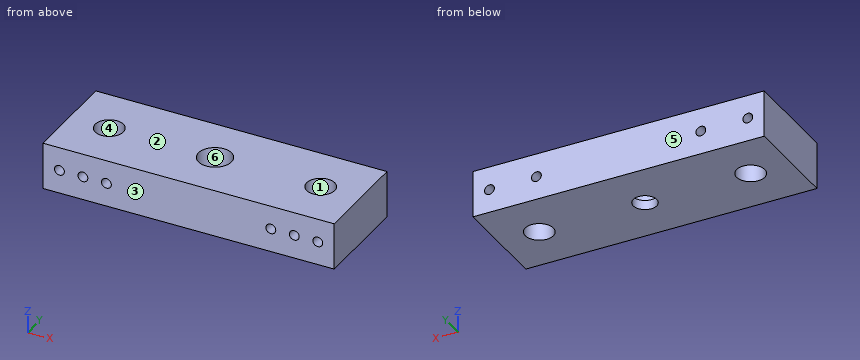
```python
from build123d import *

# Parameters (mm, degrees)
SKETCH1_W           = 124
SKETCH1_H           = 42.5
SKETCH1_R           = 6
SKETCH1_R_2         = 5
BOSS_EXTRUDE1_DEPTH = 20
CUT_EXTRUDE1_REACH  = 44.5
SKETCH2_R           = 2.1
SKETCH3_R           = 7.05
CUT_EXTRUDE2_DEPTH  = 16


with BuildPart() as part:
    # Sketch1 → Boss-Extrude1 (new body)
    with BuildSketch(Plane.XY):
        with Locations((62, 21.25)):
            Rectangle(SKETCH1_W, SKETCH1_H)
        with Locations((17, 21.25)):
            Circle(SKETCH1_R, mode=Mode.SUBTRACT)
        with Locations((107, 21.25)):
            Circle(SKETCH1_R, mode=Mode.SUBTRACT)
        with Locations((62, 21.25)):
            Circle(SKETCH1_R_2, mode=Mode.SUBTRACT)
    extrude(amount=BOSS_EXTRUDE1_DEPTH)

    # Sketch2 → Cut-Extrude1 (cut, up to next)
    with BuildSketch(Plane.XZ, mode=Mode.PRIVATE) as cut_extrude1_sk1:
        with Locations((7, 10)):
            Circle(SKETCH2_R)
    cut_extrude1_tool1 = extrude(cut_extrude1_sk1.sketch, amount=-CUT_EXTRUDE1_REACH, mode=Mode.PRIVATE) & part.part
    add(cut_extrude1_tool1.solids().sort_by_distance((7, 0, 10))[0], mode=Mode.SUBTRACT)
    # Sketch2 → Cut-Extrude1 (cut, up to next)
    with BuildSketch(Plane.XZ, mode=Mode.PRIVATE) as cut_extrude1_sk2:
        with Locations((27, 10)):
            Circle(SKETCH2_R)
    cut_extrude1_tool2 = extrude(cut_extrude1_sk2.sketch, amount=-CUT_EXTRUDE1_REACH, mode=Mode.PRIVATE) & part.part
    add(cut_extrude1_tool2.solids().sort_by_distance((27, 0, 10))[0], mode=Mode.SUBTRACT)
    # Sketch2 → Cut-Extrude1 (cut, up to next)
    with BuildSketch(Plane.XZ, mode=Mode.PRIVATE) as cut_extrude1_sk3:
        with Locations((97, 10)):
            Circle(SKETCH2_R)
    cut_extrude1_tool3 = extrude(cut_extrude1_sk3.sketch, amount=-CUT_EXTRUDE1_REACH, mode=Mode.PRIVATE) & part.part
    add(cut_extrude1_tool3.solids().sort_by_distance((97, 0, 10))[0], mode=Mode.SUBTRACT)
    # Sketch2 → Cut-Extrude1 (cut, up to next)
    with BuildSketch(Plane.XZ, mode=Mode.PRIVATE) as cut_extrude1_sk4:
        with Locations((117, 10)):
            Circle(SKETCH2_R)
    cut_extrude1_tool4 = extrude(cut_extrude1_sk4.sketch, amount=-CUT_EXTRUDE1_REACH, mode=Mode.PRIVATE) & part.part
    add(cut_extrude1_tool4.solids().sort_by_distance((117, 0, 10))[0], mode=Mode.SUBTRACT)
    # Sketch2 → Cut-Extrude1 (cut, up to next)
    with BuildSketch(Plane.XZ, mode=Mode.PRIVATE) as cut_extrude1_sk5:
        with Locations((17, 10)):
            Circle(SKETCH2_R)
    cut_extrude1_tool5 = extrude(cut_extrude1_sk5.sketch, amount=-CUT_EXTRUDE1_REACH, mode=Mode.PRIVATE) & part.part
    add(cut_extrude1_tool5.solids().sort_by_distance((17, 0, 10))[0], mode=Mode.SUBTRACT)
    # Sketch2 → Cut-Extrude1 (cut, up to next)
    with BuildSketch(Plane.XZ, mode=Mode.PRIVATE) as cut_extrude1_sk6:
        with Locations((107, 10)):
            Circle(SKETCH2_R)
    cut_extrude1_tool6 = extrude(cut_extrude1_sk6.sketch, amount=-CUT_EXTRUDE1_REACH, mode=Mode.PRIVATE) & part.part
    add(cut_extrude1_tool6.solids().sort_by_distance((107, 0, 10))[0], mode=Mode.SUBTRACT)

    # Sketch3 → Cut-Extrude2 (cut)
    with BuildSketch(Plane.XY.offset(20)):
        with Locations((62, 21.25)):
            Circle(SKETCH3_R)
    extrude(amount=-CUT_EXTRUDE2_DEPTH, mode=Mode.SUBTRACT)


solid = part.part
```
Here's how the part is built. I have some questions about the finished solid (model axes, mm). Face numbers are marked on the shaded views. A direction names the side the tool comes from. Give positions to 0.01 mm unless a question says otherwise; leave off trailing zeros. Order: outer loops, then holes, each group sorted by start corner. A loop starts at its lowest first (then second) coordinate and runs counter-clockwise, first axis right, second up. Notation, with made-up numbers: (-33.75, -16) - (19.25, -16) arc R27 ccw to (19.25, 10) - close; hole circle Ø6 at (34.25, 35.5). An arc over 180 degrees is marked (long way). Answer as a JSON object with one key per item and string values. Group by question number.
Item 1: If we section it at B-B on x = 17: Please give me the cut outline in (y, z), and give its area (3 significant figures).
Item 2: If we section it at C-C on z = 10: Give the number of separate pieces and of enclosed holes in the cut face, and give its area (3 significant figures).
Item 3: For P1, Ø7, axis at x = 63, y = 24, coming from the +Z side, with a flat end and sliding along its axis, tell me the tip position at first contact or that it passes through.
Item 4: If we section it at D-D on x = 97: Please give me the cut outline in (y, z).
Item 5: If we mould it in two halves opening along Y, with no side actions, what happens to the marked faces 1, 2, 3 and 4? For each: pulls with the +Y half, pulls with the -Y half, needs draft (parallel to the pull), parting line crosses it, or undercut.
Item 6: Which directions (+Z, -Z, +X, -X, +Y, -Y) give clear straight access to the entire face, cutting with the end or side of a thin tool? Please do the marked faces 5 and 6.
Item 7: If we section it at A-A on y = 21.25: Please give me the cut outline in (x, z), and give its area (3 significant figures).
Item 8: Please list where these lines run through material, in increasing order: probe 1 along Y at (x, z) = (62, 2.4); probe 2 along Y at (x, z) = (62, 14.5); probe 3 along X at (y, z) = (21, 6.5).
Result set:
{
 "1": {"outline": "(0, 0) - (15.25, 0) - (15.25, 7.9) - (0, 7.9) - close; (0, 12.1) - (15.25, 12.1) - (15.25, 20) - (0, 20) - close; (27.25, 0) - (42.5, 0) - (42.5, 20) - (27.25, 20) - close", "area": "546 mm²"},
 "2": {"separate pieces": "5", "enclosed holes": "1", "area": "4,040 mm²"},
 "3": {"P1": "z = 4"},
 "4": {"outline": "(0, 0) - (42.5, 0) - (42.5, 7.9) - (0, 7.9) - close; (0, 12.1) - (42.5, 12.1) - (42.5, 20) - (0, 20) - close"},
 "5": {"face 1": "undercut", "face 2": "needs draft", "face 3": "pulls with the -Y half", "face 4": "undercut"},
 "6": {"face 5": "+Z, -Z, +X, -X, +Y", "face 6": "+Z"},
 "7": {"outline": "(0, 0) - (11, 0) - (11, 20) - (0, 20) - close; (23, 0) - (57, 0) - (57, 4) - (54.95, 4) - (54.95, 20) - (23, 20) - close; (67, 0) - (101, 0) - (101, 20) - (69.05, 20) - (69.05, 4) - (67, 4) - close; (113, 0) - (124, 0) - (124, 20) - (113, 20) - close; hole circle Ø4.2 at (7, 10); hole circle Ø4.2 at (27, 10); hole circle Ø4.2 at (97, 10); hole circle Ø4.2 at (117, 10)", "area": "1,680 mm²"},
 "8": {"probe 1": "0 to 16.25, 26.25 to 42.5", "probe 2": "0 to 14.2, 28.3 to 42.5", "probe 3": "0 to 11.01, 22.99 to 54.95, 69.05 to 101.01, 112.99 to 124"}
}
